Geometry: final body of the model. Coordinates: model frame, mm. Coordinates: 2 decimals unless noted, no trailing zeros. Order: outer loops, then holes, each group sorted by start corner. A loop starts at its lowest first (then second) coordinate and runs counter-clockwise, first axis right, second up. Notation, with made-up numbers: M 67,84 L 104,84 A21 cw 104,106 Z; hole C 66,64.5 d3. An arc over 180 degrees is marked long. Use CSV: the item, a comma, the result in double quotes. Start each with the question number.
1. Section query C-C on y = 32. Return the cut outline in (x, z), and give its area (3 significant figures).
2. Material intervals for line 1 (X direction, y = 30, z = 0.6); line 2 (Y direction, x = 25.5, z = -0.9); line 3 (Y direction, x = 1.5, z = -0.05), sorted ascending.
3. Section query B-B on x = 22. Return the cut outline in (y, z), and give its area (3 significant figures).
4. Section query A-A on z = 0.1. Return the cut outline in (x, y), and give its area (3 significant figures).
5. Pull-direction query (Y, two-part tool) for faces 1 (the flat face through (-1.617, 26, 0)), 2 (the flat face through (37, 65.117, 0)), 3 (the flat face through (18, 24.347, 0)); classes: pulls with the +Y half, pulls with the -Y half, needs draft (parallel to the pull), parting line crosses it, or undercut.
Autodesk Inventor part; units mm, degrees
ref_plane "YZ Plane" through (0, 0, 0) normal (1, 0, 0) x (0, 1, 0)
ref_plane "XZ Plane" through (0, 0, 0) normal (0, 1, 0) x (-1, 0, 0)
ref_plane "XY Plane" through (0, 0, 0) normal (0, 0, 1) x (1, 0, 0)
sketch "Sketch1" plane through (0, 0, 0) normal (0, 0, 1) x (1, 0, 0)
  line L0 (39.1526, 75.1474) -> (39.1526, -26.4526)
  line L1 (-5.5514, 24.3474) -> (39.1526, 24.3474)
  line L2 (39.1526, 65.117) -> (35.1526, 65.117)
  line L3 (35.1526, 65.117) -> (-1.617, 28.3474)
  line L4 (-1.617, 28.3474) -> (-1.617, 24.3474)
  dimension "d0" = 4
  dimension "d1" = 4
  dimension "d2" = 45
  dimension "d3" = 52
extrude "Extrusion1" add sketch "Sketch1" along normal mid plane 2.5
properties part number "gusset"
Results list:
1,outline,"M 2.04,-1.25 L 39.15,-1.25 L 39.15,1.25 L 2.04,1.25 Z"
1,area,"92.8 mm²"
2,line 1,"x = 0.04 to 39.15"
2,line 2,"y = 24.35 to 55.46"
2,line 3,"y = 24.35 to 31.46"
3,outline,"M 24.35,-1.25 L 51.96,-1.25 L 51.96,1.25 L 24.35,1.25 Z"
3,area,"69.0 mm²"
4,outline,"M -1.62,24.35 L 39.15,24.35 L 39.15,65.12 L 35.15,65.12 L -1.62,28.35 Z"
4,area,"986 mm²"
5,face 1,"needs draft"
5,face 2,"pulls with the +Y half"
5,face 3,"pulls with the -Y half"
